Could you check a few things on this model? Use its own coordinates, in mm. Face numbers are marked on the shaded views. A direction names the side the tool comes from. Give positions to 0.01 mm unless a question says otherwise; leave off trailing zeros. Order: outer loops, then holes, each group sorted by start corner. A loop starts at its lowest first (then second) coordinate and runs counter-clockwise, first axis right, second up. Notation, with made-up numbers: M 15.5,63.5 L 52.5,63.5 A28 cw 52.5,88.5 Z; hole C 87,32 d8. An arc over 180 degrees is marked long. Use a Markdown table: item, result. Add a question column.
```python
from build123d import *

# Parameters (mm, degrees)
F0_W     = 38.1
F0_H     = 50.8
F1_DEPTH = 63.5
F3_DEPTH = 101.6
F4_R     = 4.7625
F5_DEPTH = 25.4


with BuildPart() as f1:
    # F0 (on Top) → F1 (new body, symmetric)
    with BuildSketch(Plane.XY):
        Rectangle(F0_W, F0_H)
    extrude(amount=F1_DEPTH, both=True)

    # F2 (on face) → F3 (cut)
    with BuildSketch(Plane(origin=(0, 0, -63.5), x_dir=(1, 0, 0), z_dir=(0, 0, -1))):
        Polygon((6.35, 25.4), (-6.35, 25.4), (-6.35, 12.7), (-19.05, 12.7), (-19.05, -12.7), (-6.35, -12.7), (-6.35, -25.4), (6.35, -25.4), (6.35, -12.7), (19.05, -12.7), (19.05, 12.7), (6.35, 12.7), align=None)
    extrude(amount=-F3_DEPTH, mode=Mode.SUBTRACT)

    # F4 (on face) → F5 (cut)
    with BuildSketch(Plane.XY.offset(63.5)):
        Circle(F4_R)
    extrude(amount=-F5_DEPTH, mode=Mode.SUBTRACT)


solid = f1.part
```
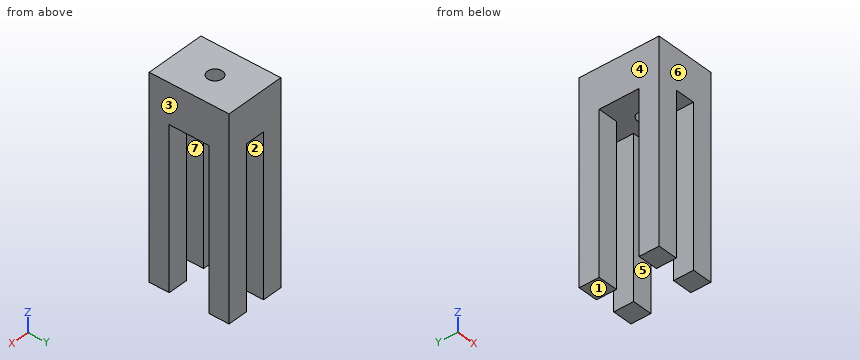
1) For the marked faces 5, 6 and 7, which set-ups out of +Z, -Z, +X, -X, +Y, -Y let a thin tool reach every point of the face, with its end or its side?
2) For pin 1 (12.5 mm diameter, centred on x = 0, y = 0, fed in from -Z), with a flat end and sliding along its axis, tell me the tip position at first contact or that it passes through.
3) Please list where these lines run through material, in increasing order: line 1 (Y direction, x = -9, z = -41); line 2 (Y direction, x = 0, z = 47); line 3 (X direction, y = 18, z = -15.5). Write a range as from..to.
4) Suppose I cut it at D-D on y = 18. Please give me the cut outline in (x, z).
5) We'd pull the mould along X, two halves only. Please class the marked faces 1, 2, 3 and 4: pulls with the +X half, pulls with the -X half, needs draft (parallel to the pull), parting line crosses it, or undercut.
6) Suppose I cut it at C-C on z = -26. Please give me the cut outline in (x, y), and give its area (3 significant figures).
7) Suppose I cut it at B-B on x = 0. Please give me the cut outline in (y, z), and give its area (3 significant figures).
8) Suppose I cut it at A-A on y = 0. Please give me the cut outline in (x, z).
Values found:
| question | item | result |
|---|---|---|
| 1 | face 5 | -Z, +X, -X |
| 1 | face 6 | +Z, -Z, +X, -X, -Y |
| 1 | face 7 | -Z, +Y, -Y |
| 2 | pin 1 | stops at z = 38.1 |
| 3 | line 1 | y = -25.4..-12.7, 12.7..25.4 |
| 3 | line 2 | y = -25.4..-4.76, 4.76..25.4 |
| 3 | line 3 | x = -19.05..-6.35, 6.35..19.05 |
| 4 | outline | M -19.05,-63.5 L -6.35,-63.5 L -6.35,38.1 L 6.35,38.1 L 6.35,-63.5 L 19.05,-63.5 L 19.05,63.5 L -19.05,63.5 Z |
| 5 | face 1 | needs draft |
| 5 | face 2 | undercut |
| 5 | face 3 | pulls with the +X half |
| 5 | face 4 | pulls with the -X half |
| 6 | outline | M -19.05,-25.4 L -6.35,-25.4 L -6.35,-12.7 L -19.05,-12.7 Z; M -19.05,12.7 L -6.35,12.7 L -6.35,25.4 L -19.05,25.4 Z; M 6.35,-25.4 L 19.05,-25.4 L 19.05,-12.7 L 6.35,-12.7 Z; M 6.35,12.7 L 19.05,12.7 L 19.05,25.4 L 6.35,25.4 Z |
| 6 | area | 645 mm^2 |
| 7 | outline | M -25.4,38.1 L -4.76,38.1 L -4.76,63.5 L -25.4,63.5 Z; M 4.76,38.1 L 25.4,38.1 L 25.4,63.5 L 4.76,63.5 Z |
| 7 | area | 1,050 mm^2 |
| 8 | outline | M -19.05,38.1 L -4.76,38.1 L -4.76,63.5 L -19.05,63.5 Z; M 4.76,38.1 L 19.05,38.1 L 19.05,63.5 L 4.76,63.5 Z |
